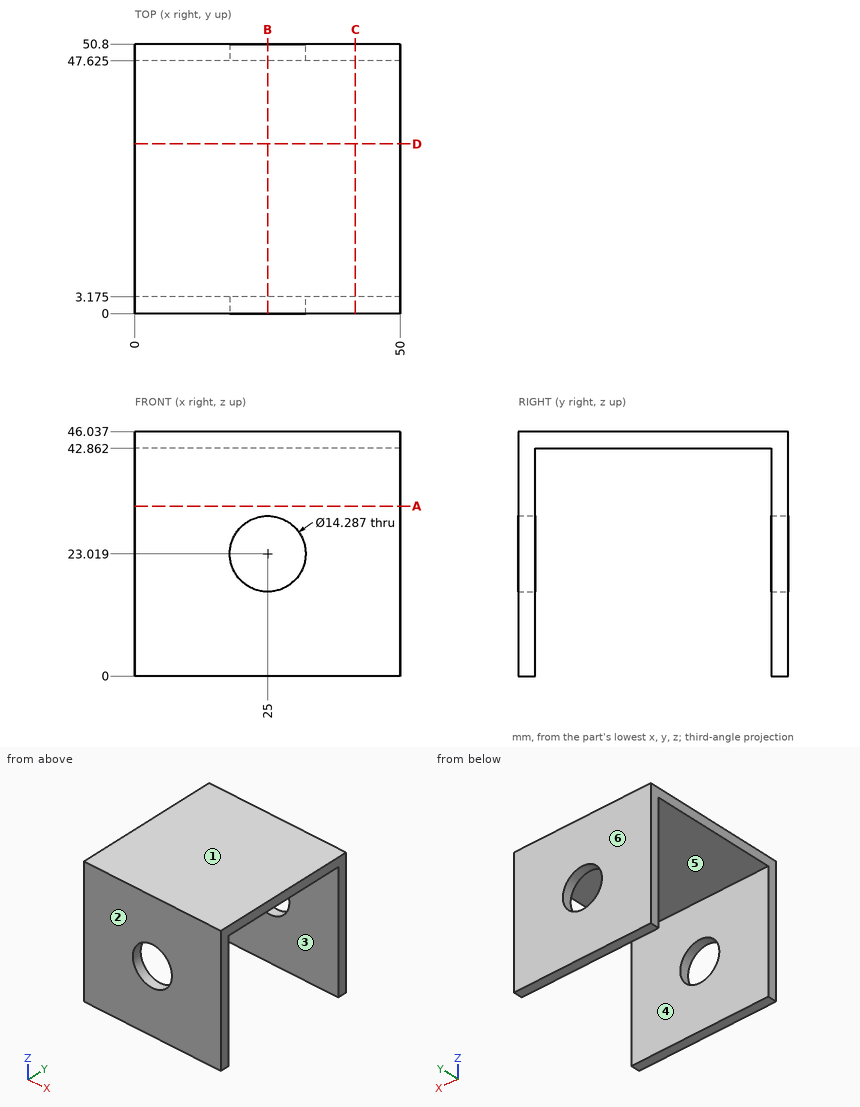
Could you check a few things on this drawing? It's one solid part, dimensions in mm from its lowest x, y, z. A direction names the side the tool comes from. Coordinates: 2 decimals unless noted, no trailing zeros. Write each loop counter-clockwise with the first axis right and the second up, starting at its lowest first coordinate (ties: lowest second). Pieces come first, ordered by that corner, then holes.
1) If I drill on line 1 (Y direction, x = 43.5, z = 25) (1 decimal); line 2 (Z direction, x = 25, y = 49.2) (1 decimal); line 3 (Z direction, x = 46.5, y = 16), over which ranges is the centre line in solid material (lowest first)?
Filled in:
line 1: y = 0 to 3.2, 47.6 to 50.8
line 2: z = 0 to 15.9, 30.2 to 46
line 3: z = 42.86 to 46.04
2) I'm going to push flat-ended pins straight in: pin 1 (12 mm diameter, centred on x = 28.5, y = 17.5, fed in from -Z); pin 2 (8.5 mm diameter, centred on x = 25, z = 23.02, fed in from -Y); pin 3 (23 mm diameter, centred on x = 25, z = 23.02, fed in from -Y). Where does each tip first touch, or does it pass through?
Filled in:
pin 1: stops at z = 42.86
pin 2: passes through
pin 3: stops at y = 0
3) If we section it at B-B (x = 25): List the corners of the cut face in (y, z) for me (1 decimal), plus the area to 3 significant figures.
Filled in:
outline: (0, 0) - (3.2, 0) - (3.2, 15.9) - (0, 15.9) - close; (0, 30.2) - (3.2, 30.2) - (3.2, 42.9) - (47.6, 42.9) - (47.6, 30.2) - (50.8, 30.2) - (50.8, 46) - (0, 46) - close; (47.6, 0) - (50.8, 0) - (50.8, 15.9) - (47.6, 15.9) - close
area: 343 mm2
4) Thinking about a two-plate mould opening in Y: for the marked faces 1, 2, 3 and 4, which applies, +Y half, -Y half, draft (parallel to the pull), parting line (faces both ways), or undercut?
Filled in:
face 1: draft
face 2: -Y half
face 3: undercut
face 4: undercut
5) If we section it at C-C (x = 41.5): List the corners of the cut face in (y, z) for me (1 decimal).
Filled in:
outline: (0, 0) - (3.2, 0) - (3.2, 42.9) - (47.6, 42.9) - (47.6, 0) - (50.8, 0) - (50.8, 46) - (0, 46) - close
6) Which directions (+Z, -Z, +X, -X, +Y, -Y) give clear straight access to the entire face, cutting with the end or side of a thin tool? Please do the marked faces 5 and 6.
Filled in:
face 5: -Z, +X, -X
face 6: +Z, -Z, +X, -X, +Y
7) If we section it at A-A (z = 32): List the corners of the cut face in (x, y) for me (1 decimal).
Filled in:
outline: (0, 0) - (50, 0) - (50, 3.2) - (0, 3.2) - close; (0, 47.6) - (50, 47.6) - (50, 50.8) - (0, 50.8) - close
8) If we section it at D-D (y = 32): List the corners of the cut face in (x, z) for me.
Filled in:
outline: (0, 42.86) - (50, 42.86) - (50, 46.04) - (0, 46.04) - close
